from build123d import *

# Parameters (mm, degrees)
SKETCH1_W           = 46.55
SKETCH1_H           = 2
BOSS_EXTRUDE1_DEPTH = 2
SKETCH11_W          = 46.55
SKETCH11_H          = 37.66
BOSS_EXTRUDE3_DEPTH = 2
SKETCH12_R          = 1.27
CUT_EXTRUDE6_DEPTH  = 2


with BuildPart() as part:
    # Sketch1 → Boss-Extrude1 (new body)
    with BuildSketch(Plane.XY):
        with Locations((-25.275, 40.66)):
            Rectangle(SKETCH1_W, SKETCH1_H)
        Polygon((-2, 0), (0, 0), (0, 41.66), (-2, 41.66), (-2, 39.66), (-2, 2), align=None)
        Polygon((-50.55, 0), (-48.55, 0), (-48.55, 2), (-48.55, 39.66), (-48.55, 41.66), (-50.55, 41.66), align=None)
        with Locations((-25.275, 1)):
            Rectangle(SKETCH1_W, SKETCH1_H)
    extrude(amount=BOSS_EXTRUDE1_DEPTH)

    # Sketch11 → Boss-Extrude3 (add)
    with BuildSketch(Plane(origin=(0, 0, 0), x_dir=(-1, 0, 0), z_dir=(0, 0, -1))):
        with Locations((25.275, 20.83)):
            Rectangle(SKETCH11_W, SKETCH11_H)
    extrude(amount=-BOSS_EXTRUDE3_DEPTH)

    # Sketch12 → Cut-Extrude6 (cut)
    with BuildSketch(Plane(origin=(0, 0, 0), x_dir=(-1, 0, 0), z_dir=(0, 0, -1))):
        with Locations((2.59, 39.07)):
            Circle(SKETCH12_R)
        with Locations((47.96, 39.07)):
            Circle(SKETCH12_R)
        with Locations((2.59, 2.59)):
            Circle(SKETCH12_R)
        with Locations((47.96, 2.59)):
            Circle(SKETCH12_R)
    extrude(amount=-CUT_EXTRUDE6_DEPTH, mode=Mode.SUBTRACT)


solid = part.part
Could you check a few things on this model? Use its own coordinates, in mm. Round coordinates to 2 decimals unless told otherwise and drop trailing zeros. Write each loop counter-clockwise with the first axis right and the second up, starting at its lowest first coordinate (ties: lowest second). Pieces come first, ordered by that corner, then holes. Notation, with made-up numbers: (84, 87.5) - (138, 87.5) arc R18 ccw to (138, 100.5) - close; hole circle Ø3 at (39.5, 81.5). An arc over 180 degrees is marked (long way). Put each result on its own line as item: value. Start each with the question number.
(1) Will this pin go through, and if not, where does the flat tip stop? pin 1 (1.5 mm diameter, centred on x = -47.96, y = 2.59, fed in from +Z).
(2) Thinking about a two-plate mould opening in Y: for faces 1 (the flat face through (-26, 0, 1)), 2 (the cylindrical face through (-2.31, 37.83, 0.99)), 3 (the flat face through (-25, 41.66, 1)), 4 (the flat face through (0, 21, 1)), which applies, released by +Y, released by -Y, zero draft, split by the parting line, or undercut?
(3) I want a section at A-A, the plane x = -47.96. Please give me the cut outline in (y, z), plus the area to 3 significant figures.
(4) I want a section at B-B, the plane y = 39.07. Please give me the cut outline in (x, z), plus the area to 3 significant figures.
(5) I need wall thicknesses on probe 1 along Y at (x, z) = (-47.96, 1.6); probe 2 along X at (y, z) = (3.5, 1.9); probe 3 along Y at (x, z) = (-47, 0.2). Which ranges of each line are inside material? Lowest first, please.
Here are the results:
1. pin 1: passes through
2. face 1: released by -Y
2. face 2: undercut
2. face 3: released by +Y
2. face 4: zero draft
3. outline: (0, 0) - (1.32, 0) - (1.32, 2) - (0, 2) - close; (3.86, 0) - (37.8, 0) - (37.8, 2) - (3.86, 2) - close; (40.34, 0) - (41.66, 0) - (41.66, 2) - (40.34, 2) - close
3. area: 73.2 mm^2
4. outline: (-50.55, 0) - (-49.23, 0) - (-49.23, 2) - (-50.55, 2) - close; (-46.69, 0) - (-3.86, 0) - (-3.86, 2) - (-46.69, 2) - close; (-1.32, 0) - (0, 0) - (0, 2) - (-1.32, 2) - close
4. area: 90.9 mm^2
5. probe 1: y = 0 to 1.32, 3.86 to 37.8, 40.34 to 41.66
5. probe 2: x = -50.55 to -48.85, -47.07 to -3.48, -1.7 to 0
5. probe 3: y = 0 to 1.76, 3.42 to 38.24, 39.9 to 41.66
